Check sheet for the modelled part. Datum: model origin and axes. Units: mm. A direction names the side the tool comes from. Round coordinates to 2 decimals unless told otherwise and drop trailing zeros. Order: outer loops, then holes, each group sorted by start corner. A loop starts at its lowest first (then second) coordinate and runs counter-clockwise, first axis right, second up.
(1) Sectioned sample at B-B, the plane y = -5.75. Count the separate pieces of the cut face and the enclosed holes in it, and give its area (3 significant figures).
(2) Thickness scan on probe 1 along Z at (x, y) = (97.5, -2.25); probe 2 along X at (y, z) = (-4, 57.5); probe 3 along X at (y, z) = (-4.5, 6). Record the ranges inside material, lowest first.
(3) Mould release check, pull along X, two halves, no side actions. Record for faces 6 (the flat face through (52, -5, 70)), 7 (the cylindrical face through (26.284, -5.69, 52.685)), 8 (the cylindrical face through (92.65, -0.41, 50)): released by +X, released by -X, zero draft, split by the parting line, or undercut.
(4) Tool access check on faces 1 (the flat face through (95.8, -0.8, 44.9)), 2 (the flat face through (53.8, 1, 50)), 3 (the flat face through (51, 1, 40)), 4 (the flat face through (48.8, 1, 50)), 5 (the cylindrical face through (46.3, -0.76, 22.55)). Record the directions out of +Z, -Z, +X, -X, +Y, -Y that give a thin tool (end or side, any length) a straight path to the whole face; none if there is none.
(5) Sectioned sample at D-D, the plane x = 97.5. Enter the section's corners in (y, z), and give its area (3 significant figures).
(6) Depth check by flat-ended pin: pin 1 (7 mm diameter, centred on x = 10, z = 57.5, fed in from +Y); pin 2 (3 mm diameter, centred on x = 97.6, z = 45, fed in from +Y); pin 3 (0.8 mm diameter, centred on x = 1.5, y = 0.5, fed in from +Z); pin 4 (1.2 mm diameter, centred on x = 78, y = 2, fed in from -Z). Enter the tip coordinate at first touch or a pass-through.
(7) Sectioned sample at A-A, the plane x = 27.5. Enter the section's corners in (y, z).
(8) Sectioned sample at C-C, the plane z = 63.8. Enter the section's corners in (x, y).
Autodesk Fusion 360 part; units mm, degrees
sketch "Skizze1" plane through (0, 0, 0) normal (0, 1, 0) x (1, 0, 0)
  line L0 (0, 0) -> (102.5, 0)
  line L1 (102.5, 0) -> (102.5, -70)
  line L2 (102.5, -70) -> (0, -70)
  line L3 (0, -70) -> (0, 0)
  line L4 (0, 0) -> (5, 0)
  line L5 (5, 0) -> (5, -25)
  line L6 (5, -25) -> (0, -25)
  line L7 (0, -25) -> (0, 0)
  line L8 (0, 0) -> (25, 0)
  line L9 (25, 0) -> (25, -7.5)
  line L10 (25, -7.5) -> (0, -7.5)
  line L11 (0, -7.5) -> (0, 0)
  circle A0 centre (5, -7.5) radius 4
  circle A1 centre (27.5, -53.8) radius 1.65
  circle A2 centre (51.3, -27.5) radius 1.65
  line L12 (55.1, -25.926) -> (52.874, -23.7)
  line L13 (52.874, -23.7) -> (49.726, -23.7)
  line L14 (49.726, -23.7) -> (47.5, -25.926)
  line L15 (47.5, -25.926) -> (47.5, -29.074)
  line L16 (47.5, -29.074) -> (49.726, -31.3)
  line L17 (49.726, -31.3) -> (52.874, -31.3)
  line L18 (52.874, -31.3) -> (55.1, -29.074)
  line L19 (55.1, -29.074) -> (55.1, -25.926)
  line L20 (31.3, -52.226) -> (29.074, -50)
  line L21 (29.074, -50) -> (25.926, -50)
  line L22 (25.926, -50) -> (23.7, -52.226)
  line L23 (23.7, -52.226) -> (23.7, -55.374)
  line L24 (23.7, -55.374) -> (25.926, -57.6)
  line L25 (25.926, -57.6) -> (29.074, -57.6)
  line L26 (29.074, -57.6) -> (31.3, -55.374)
  line L27 (31.3, -55.374) -> (31.3, -52.226)
  line L28 (57.3, -21.5) -> (45.3, -21.5)
  line L29 (45.3, -21.5) -> (45.3, -33.5)
  line L30 (45.3, -33.5) -> (57.3, -33.5)
  line L31 (57.3, -33.5) -> (57.3, -21.5)
  line L32 (57.3, -21.5) -> (45.3, -33.5) construction
  line L33 (45.3, -21.5) -> (57.3, -33.5) construction
  line L34 (33.5, -47.8) -> (21.5, -47.8)
  line L35 (21.5, -47.8) -> (21.5, -59.8)
  line L36 (21.5, -59.8) -> (33.5, -59.8)
  line L37 (33.5, -59.8) -> (33.5, -47.8)
  line L38 (33.5, -47.8) -> (21.5, -59.8) construction
  line L39 (21.5, -47.8) -> (33.5, -59.8) construction
  circle A3 centre (55, -7.5) radius 3
  circle A4 centre (10, -57.5) radius 3
  line L40 (48.8, -40) -> (53.8, -40)
  line L41 (53.8, -40) -> (53.8, -60)
  line L42 (53.8, -60) -> (48.8, -60)
  line L43 (48.8, -60) -> (48.8, -40)
  line L44 (63.8, -12.5) -> (93.8, -12.5)
  line L45 (93.8, -12.5) -> (93.8, -20)
  line L46 (93.8, -20) -> (63.8, -20)
  line L47 (63.8, -20) -> (63.8, -12.5)
  line L48 (77.226, -60) -> (75, -62.226)
  circle A5 centre (78.8, -63.8) radius 1.65
  line L49 (75, -65.374) -> (77.226, -67.6)
  line L50 (80.374, -67.6) -> (82.6, -65.374)
  line L51 (72.8, -57.55) -> (72.8, -70.05)
  line L52 (75, -62.226) -> (75, -65.374)
  line L53 (84.8, -70.05) -> (84.8, -57.55)
  line L54 (84.8, -57.55) -> (72.8, -57.55)
  line L55 (72.8, -57.55) -> (84.8, -70.05) construction
  line L56 (82.6, -62.226) -> (80.374, -60)
  line L57 (77.226, -67.6) -> (80.374, -67.6)
  line L58 (80.374, -60) -> (77.226, -60)
  line L59 (82.6, -65.374) -> (82.6, -62.226)
  line L60 (72.8, -70.05) -> (84.8, -70.05)
  line L61 (84.8, -57.55) -> (72.8, -70.05) construction
  line L62 (96.026, -41.2) -> (93.8, -43.426)
  circle A6 centre (97.6, -45) radius 1.65
  line L63 (93.8, -46.574) -> (96.026, -48.8)
  line L64 (99.174, -48.8) -> (101.4, -46.574)
  line L65 (91.6, -39) -> (91.6, -51)
  line L66 (93.8, -43.426) -> (93.8, -46.574)
  line L67 (103.6, -51) -> (103.6, -39)
  line L68 (103.6, -39) -> (91.6, -39)
  line L69 (91.6, -39) -> (103.6, -51) construction
  line L70 (101.4, -43.426) -> (99.174, -41.2)
  line L71 (96.026, -48.8) -> (99.174, -48.8)
  line L72 (99.174, -41.2) -> (96.026, -41.2)
  line L73 (101.4, -46.574) -> (101.4, -43.426)
  line L74 (91.6, -51) -> (103.6, -51)
  line L75 (103.6, -39) -> (91.6, -51) construction
  line L76 (42.5, -15) -> (12.5, -15)
  line L77 (12.5, -15) -> (12.5, -45)
  line L78 (12.5, -45) -> (42.5, -45)
  line L79 (42.5, -45) -> (42.5, -15)
  line L80 (42.5, -15) -> (12.5, -45) construction
  line L81 (12.5, -15) -> (42.5, -45) construction
  circle A7 centre (41, -57.5) radius 3
  circle A8 centre (97.5, -7.5) radius 3
  point P0 (51.3, -27.5)
  point P1 (27.5, -53.8)
  point P2 (51.3, -27.5)
  point P3 (27.5, -53.8)
  point P4 (78.8, -63.8)
  point P5 (78.8, -63.8)
  point P6 (97.6, -45)
  point P7 (97.6, -45)
  point P8 (27.5, -30)
  dimension "d1" = 102.5
  dimension "d2" = 70
  dimension "d3" = 5
  dimension "d4" = 25
  dimension "d5" = 25
  dimension "d6" = 7.5
  dimension "d7" = 8
  dimension "d8" = 3.3
  dimension "d9" = 46.3
  dimension "d11" = 3.3
  dimension "d13" = 46.3
  dimension "d14" = 20
  dimension "d15" = 22.5
  dimension "d16" = 3.8
  dimension "d17" = 3.8
  dimension "d18" = 12
  dimension "d19" = 12
  dimension "d20" = 12
  dimension "d21" = 12
  dimension "d34" = 6
  dimension "d35" = 6
  dimension "d36" = 7.5
  dimension "d37" = 55
  dimension "d38" = 50
  dimension "d39" = 10
  dimension "d40" = 5
  dimension "d41" = 20
  dimension "d42" = 2.5
  dimension "d43" = 60
  dimension "d44" = 30
  dimension "d45" = 7.5
  dimension "d47" = 10
  dimension "d48" = 3.3
  dimension "d49" = 3.8
  dimension "d50" = 12
  dimension "d51" = 12.5
  dimension "d52" = 43.8
  dimension "d53" = 15
  dimension "d54" = 3.3
  dimension "d55" = 3.8
  dimension "d56" = 12
  dimension "d57" = 12
  dimension "d58" = 43.8
  dimension "d59" = 15
  dimension "d84" = 20
  dimension "d85" = 30
  dimension "d86" = 30
  dimension "d87" = 22.5
  dimension "d88" = 22.5
  dimension "d131" = 6
  dimension "d132" = 50
  dimension "d133" = 31
  dimension "d134" = 6
  dimension "d135" = 7.5
  dimension "d136" = 5
extrude "Extrusion1" add sketch "Skizze1" against normal blind 10 contours L0 L3 L4 L5 L7 L8 L10 L11 A0 | L0 L5 L8 L9 L10 A0 | L3 L5 L6 L7 L10 A0 | L0 L1 L2 L3 L5 L6 L9 L10 A0 L51 L53 L54 L65 L68 L74 | L5 L10 A0 | L5 L10 A0 | L5 L10 A0 | L5 L10 A0 | L1 L65 L68 L74 | L2 L51 L53 L54 | L12 L13 L14 L15 L16 L17 L18 L19 | L20 L21 L22 L23 L24 L25 L26 L27 | L28 L29 L30 L31 | L34 L35 L36 L37 | L40 L41 L42 L43 | L44 L45 L46 L47 | L48 L49 L50 L52 L56 L57 L58 L59 | L62 L63 L64 L66 L70 L71 L72 L73 | L76 L77 L78 L79 makes body 1
extrude "Extrusion2" add sketch "Skizze1" along normal blind 1.5 contours L0 L3 L4 L5 L7 L8 L10 L11 A0 | L0 L5 L8 L9 L10 A0 | L3 L5 L6 L7 L10 A0 bodies 1
extrude "Extrusion3" cut sketch "Skizze1" against normal blind 1.5 contours A1 | A2 | L12 L13 L14 L15 L16 L17 L18 L19 | L20 L21 L22 L23 L24 L25 L26 L27 | L28 L29 L30 L31 | L34 L35 L36 L37 | L76 L77 L78 L79 bodies 1
extrude "Extrusion5" add sketch "Skizze1" along normal blind 2.5 contours L40 L41 L42 L43 | L44 L45 L46 L47 bodies 1
extrude "Extrusion6" cut sketch "Skizze1" against normal blind 0.8 contours L1 L67 L68 L74 | L1 L65 L68 L74 | L2 L51 L53 L54 | L2 L51 L53 L60 | L48 L49 L50 L52 L56 L57 L58 L59 | L62 L63 L64 L66 L70 L71 L72 L73 bodies 1
fillet "Abrundung1" radius 3.5 10 edges at (21.5, -0.75, 59.8) (45.3, -0.75, 33.5) (57.3, -0.75, 33.5) (33.5, -0.75, 59.8) (57.3, -0.75, 21.5) (33.5, -0.75, 47.8) (45.3, -0.75, 21.5) (21.5, -0.75, 47.8) (9, 0.75, 7.5) (5, 0.75, 11.5) on bodies 1
fillet "Abrundung1" radius 3.5 7 edges at (42.5, -0.75, 15) (42.5, -0.75, 45) (12.5, -0.75, 45) (12.5, -0.75, 15) (72.8, -0.4, 57.55) (91.6, -0.4, 39) (84.8, -0.4, 57.55) on bodies 1
fillet "Abrundung1" radius 3.5 1 edges at (91.6, -0.4, 51) on bodies 1
copy_body "Körper->Berechn1" bodies 1 removing the originals makes body 2 in component "Fixture"
component "Fixture" placed x (1, 0, 0) y (0, 1, 0) z (0, 0, 1) at (0, 0, 0)
equation "d9 = 3.8 mm + 42.5 mm"
equation "d13 = d9"
equation "d52 = 40 mm + 3.8 mm"
equation "d58 = d52"
equation "d62 = -2.8 mm + 2 mm"
equation "d132 = d38"
Derived:
1. separate pieces: 1
1. enclosed holes: 8
1. area: 7,030 mm2
2. probe 1: z = 0 to 4.5, 10.5 to 43.35, 46.65 to 70
2. probe 2: x = 0 to 7, 13 to 38, 44 to 102.5
2. probe 3: x = 0 to 52.4, 57.6 to 94.9, 100.1 to 102.5
3. face 6: zero draft
3. face 7: undercut
3. face 8: released by +X
4. face 1: +X, +Y
4. face 2: +Z, -Z, +X, +Y
4. face 3: -Z, +X, -X, +Y
4. face 4: +Z, -Z, -X, +Y
4. face 5: +Y
5. outline: (-10, 0) - (0, 0) - (0, 4.5) - (-10, 4.5) - close; (-10, 10.5) - (0, 10.5) - (0, 39) - (-0.8, 39) - (-0.8, 43.35) - (-10, 43.35) - close; (-10, 46.65) - (-0.8, 46.65) - (-0.8, 51) - (0, 51) - (0, 70) - (-10, 70) - close
5. area: 600 mm2
6. pin 1: stops at y = 0
6. pin 2: passes through
6. pin 3: stops at z = 25
6. pin 4: stops at z = 12.5
7. outline: (-10, 0) - (0, 0) - (0, 15) - (-1.5, 15) - (-1.5, 45) - (0, 45) - (0, 47.8) - (-1.5, 47.8) - (-1.5, 52.15) - (-10, 52.15) - close; (-10, 55.45) - (-1.5, 55.45) - (-1.5, 59.8) - (0, 59.8) - (0, 70) - (-10, 70) - close
8. outline: (0, -10) - (77.15, -10) - (77.15, -0.8) - (72.8, -0.8) - (72.8, 0) - (0, 0) - close; (80.45, -10) - (102.5, -10) - (102.5, 0) - (84.8, 0) - (84.8, -0.8) - (80.45, -0.8) - close
